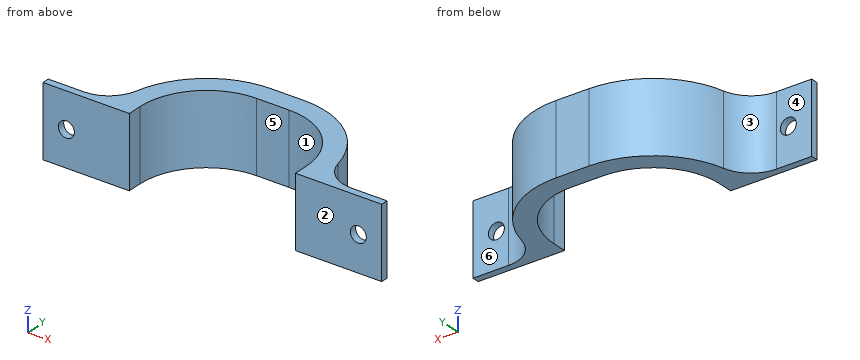
```python
from build123d import *

# Parameters (mm, degrees)
F1_DEPTH = 20
F3_D     = 4.5
F4_D     = 4.5
F5_DEPTH = 2
F6_DEPTH = 2


with BuildPart() as f1:
    # F0 (on Top) → F1 (new body)
    with BuildSketch(Plane.XY):
        with BuildLine():
            Line((-37.8199822518, -7.4723315098), (-45.8199822518, -7.4723315098))
            Line((-45.8199822518, -7.4723315098), (-45.8199822518, -9.4723315098))
            Line((-45.8199822518, -9.4723315098), (-28.8447495745, -9.4723315098))
            Line((-28.8447495745, -9.4723315098), (-23.45, -9.4723315098))
            Line((-23.45, -9.4723315098), (-23.45, -7.887919838))
            Line((-23.45, -7.887919838), (-23.45, -5.3745856304))
            ThreePointArc((-23.45, -5.3745856304), (-17.9429472697, 7.9206157599), (-4.6477458794, 13.4276684902))
            Line((-4.6477458794, 13.4276684902), (0, 13.4276684902))
            Line((0, 13.4276684902), (4.6477458794, 13.4276684902))
            ThreePointArc((4.6477458794, 13.4276684902), (17.9429472697, 7.9206157599), (23.45, -5.3745856304))
            Line((23.45, -5.3745856304), (23.45, -7.887919838))
            Line((23.45, -7.887919838), (23.45, -9.4723315098))
            Line((23.45, -9.4723315098), (28.8447495745, -9.4723315098))
            Line((28.8447495745, -9.4723315098), (45.8199822518, -9.4723315098))
            Line((45.8199822518, -9.4723315098), (45.8199822518, -7.4723315098))
            Line((45.8199822518, -7.4723315098), (37.8199822518, -7.4723315098))
            ThreePointArc((37.8199822518, -7.4723315098), (31.8371692612, -5.3745856304), (28.4743700766, 0))
            ThreePointArc((28.4743700766, 0), (19.9009167747, 13.7024940459), (4.6477458794, 19.0506920822))
            Line((4.6477458794, 19.0506920822), (0, 19.0506920822))
            Line((0, 19.0506920822), (-4.6477458794, 19.0506920822))
            ThreePointArc((-4.6477458794, 19.0506920822), (-19.9009167747, 13.7024940459), (-28.4743700766, 0))
            ThreePointArc((-28.4743700766, 0), (-31.8371692612, -5.3745856304), (-37.8199822518, -7.4723315098))
        make_face()
    extrude(amount=F1_DEPTH)

    # F3 (through all)
    with Locations(Plane(origin=(0, -7.4723315098, 0), x_dir=(-1, 0, 0), z_dir=(0, 1, 0))):
        with Locations((-41.2173499218, 10)):
            Hole(F3_D / 2)

    # F4 (through all)
    with Locations(Plane(origin=(0, -7.4723315098, 0), x_dir=(-1, 0, 0), z_dir=(0, 1, 0))):
        with Locations((41.2173499218, 10)):
            Hole(F4_D / 2)

    # F5 (add): a face of the model
    f5_faces = [f1.faces().sort_by_distance(p)[0] for p in [
        (-45.8199822518, -8.4723315098, 10),
    ]]
    extrude(f5_faces, amount=F5_DEPTH)

    # F6 (add): a face of the model
    f6_faces = [f1.faces().sort_by_distance(p)[0] for p in [
        (45.8199822518, -8.4723315098, 10),
    ]]
    extrude(f6_faces, amount=F6_DEPTH)


solid = f1.part
```
Check sheet for the modelled part. Datum: model origin and axes. Units: mm. Face numbers are marked on the shaded views. A direction names the side the tool comes from. Give positions to 0.01 mm unless a question says otherwise; leave off trailing zeros. Write each loop counter-clockwise with the first axis right and the second up, starting at its lowest first coordinate (ties: lowest second). Pieces come first, ordered by that corner, then holes. Notation, with made-up numbers: (67, 41.5) - (109, 41.5) arc R20 cw to (109, 66.5) - close; hole circle Ø7 at (25, 27). An arc over 180 degrees is marked (long way). Answer as a JSON object with one key per item and string values. Group by question number.
1) Thickness scan on probe 1 along X at (y, z) = (-8.5, 18.75); probe 2 along X at (y, z) = (-2.5, 18.75); probe 3 along Y at (x, z) = (11.5, 5.5). Record the ranges inside material, lowest first. Write a range as from..to.
2) Sectioned sample at C-C (z = 6.25). Record the cut outline in (x, y).
3) Depth check by flat-ended pin: P1, Ø7.5, axis at x = 2, z = 9, coming from the -Y side; P2, Ø11, axis at x = -43.5, z = 7, coming from the +Y side; P3, Ø3, axis at y = 11, z = 16.5, coming from the -X side. Enter the tip coordinate at first touch or a pass-through.
4) Sectioned sample at B-B (y = 9.5). Record the cut outline in (x, z), then the cut area to 3 significant figures.
5) Sectioned sample at A-A (z = 10). Record the cut outline in (x, y), then the cut area to 3 significant figures.
6) Access from +Z, -Z, +X, -X, +Y, -Y to the whole of each face (thin tool, end or side, straight path). Record for the marked faces 4, 5 and 6.
7) Release check for a two-part mould opening along X. For the marked faces 1, 2 and 3 record: pulls with the +X half, pulls with the -X half, needs draft (parallel to the pull), parting line crosses it, or undercut.
8) Sectioned sample at D-D (x = -3.5). Record the cut outline in (y, z), then the cut area to 3 significant figures.
Geometry results:
{
 "1": {"probe 1": "x = -47.82..-23.45, 23.45..47.82", "probe 2": "x = -29.42..-23.23, 23.23..29.42", "probe 3": "y = 12.13..18.07"},
 "2": {"outline": "(-47.82, -9.47) - (-23.45, -9.47) - (-23.45, -5.37) arc R18.8 cw to (-4.65, 13.43) - (4.65, 13.43) arc R18.8 cw to (23.45, -5.37) - (23.45, -9.47) - (47.82, -9.47) - (47.82, -7.47) - (37.82, -7.47) arc R9.58 cw to (28.47, 0) arc R24.43 ccw to (4.65, 19.05) - (-4.65, 19.05) arc R24.43 ccw to (-28.47, 0) arc R9.58 cw to (-37.82, -7.47) - (-47.82, -7.47) - close"},
 "3": {"P1": "stops at y = 13.4", "P2": "stops at y = -7.47", "P3": "stops at x = -24.02"},
 "4": {"outline": "(-24.02, 0) - (-16.15, 0) - (-16.15, 20) - (-24.02, 20) - close; (16.15, 0) - (24.02, 0) - (24.02, 20) - (16.15, 20) - close", "area": "315 mm^2"},
 "5": {"outline": "(-47.82, -9.47) - (-43.47, -9.47) - (-43.47, -7.47) - (-47.82, -7.47) - close; (-38.97, -9.47) - (-23.45, -9.47) - (-23.45, -5.37) arc R18.8 cw to (-4.65, 13.43) - (4.65, 13.43) arc R18.8 cw to (23.45, -5.37) - (23.45, -9.47) - (38.97, -9.47) - (38.97, -7.47) - (37.82, -7.47) arc R9.58 cw to (28.47, 0) arc R24.43 ccw to (4.65, 19.05) - (-4.65, 19.05) arc R24.43 ccw to (-28.47, 0) arc R9.58 cw to (-37.82, -7.47) - (-38.97, -7.47) - close; (43.47, -9.47) - (47.82, -9.47) - (47.82, -7.47) - (43.47, -7.47) - close", "area": "566 mm^2"},
 "6": {"face 4": "+Z, -Z, -X, +Y", "face 5": "+Z, -Z, -Y", "face 6": "+Z, -Z, +X, +Y"},
 "7": {"face 1": "undercut", "face 2": "needs draft", "face 3": "pulls with the -X half"},
 "8": {"outline": "(13.43, 0) - (19.05, 0) - (19.05, 20) - (13.43, 20) - close", "area": "112 mm^2"}
}
